Autodesk Inventor part; units mm, degrees
ref_plane "YZ Plane" through (0, 0, 0) normal (1, 0, 0) x (0, 1, 0)
ref_plane "XZ Plane" through (0, 0, 0) normal (0, 1, 0) x (-1, 0, 0)
ref_plane "XY Plane" through (0, 0, 0) normal (0, 0, 1) x (1, 0, 0)
sketch "Sketch1" plane through (0, 0, 0) normal (0, 0, 1) x (1, 0, 0)
  line L0 (-86, -45) -> (-46.4758, -45)
  arc A0 (-46.4758, -45) -> (-36.6914, -26.0526) centre (-46.4758, -33) ccw
  arc A1 (36.6914, -26.0526) -> (-36.6914, -26.0526) centre (0, 0) ccw
  arc A2 (36.6914, -26.0526) -> (46.4758, -45) centre (46.4758, -33) ccw
  line L1 (46.4758, -45) -> (86, -45)
  line L2 (0, -90.5431) -> (0, 67.5905) construction
  line L3 (-86, -61) -> (-46.4758, -61)
  arc A3 (-46.4758, -61) -> (-23.6456, -16.7895) centre (-46.4758, -33) ccw
  arc A4 (23.6456, -16.7895) -> (-23.6456, -16.7895) centre (0, 0) ccw
  arc A5 (23.6456, -16.7895) -> (46.4758, -61) centre (46.4758, -33) ccw
  line L4 (46.4758, -61) -> (86, -61)
  line L5 (-86, -45) -> (-86, -61)
  line L6 (86, -45) -> (86, -61)
  dimension "d0" = 90
  dimension "d1" = 12
  dimension "d2" = 45
  dimension "d3" = 172
  dimension "d4" = 16
extrude "Extrusion1" add sketch "Sketch1" along normal mid plane 70
sketch "Sketch2" plane through (0, 0, 0) normal (1, 0, 0) x (0, 1, 0)
  arc A0 (6.3443, 4) -> (6.3443, -4) centre (0, 0) ccw
  line L0 (6.3443, 4) -> (45, 4)
  line L1 (45, 4) -> (45, -4)
  line L2 (45, -4) -> (6.3443, -4)
  line L3 (45, -35) -> (45, 35)
  dimension "d7" = 15
  dimension "d8" = 8
extrude "Extrusion2" cut sketch "Sketch2" along normal through all both and the other way through all
sketch "Sketch3" plane through (0, 0, 0) normal (0, 0, 1) x (1, 0, 0)
  arc A0 (0, 73) -> (0, 17) centre (0, 45) ccw
  line L0 (-86, -61) -> (-46.4758, -61)
  line L1 (0, 73) -> (0, 17)
  arc A1 (44.5505, 6.3443) -> (-44.5505, 6.3443) centre (0, 0) ccw
  point P0 (-66.2379, -61)
  point P1 (0, 45)
  dimension "d11" = 28
  dimension "d12" = 106
revolve "Revolution1" cut sketch "Sketch3" angle 360 about axis through (0, 73, 0) along (0, -1, 0)
sketch "Sketch4" plane through (46.4758, -45, 35) normal (0, 1, 0) x (1, 0, 0)
  line L0 (18.5242, 19) -> (18.5242, 51) construction
  line L1 (12.5242, 19) -> (12.5242, 51)
  line L2 (24.5242, 51) -> (24.5242, 19)
  arc A0 (12.5242, 19) -> (24.5242, 19) centre (18.5242, 19) ccw
  arc A1 (24.5242, 51) -> (12.5242, 51) centre (18.5242, 51) ccw
  point P0 (-46.4758, 35)
  point P1 (18.5242, 35)
  dimension "d14" = 6
  dimension "d15" = 32
  dimension "d16" = 65
extrude "Extrusion3" cut sketch "Sketch4" against normal through all
mirror "Mirror1" about plane through (0, 0, 0) normal (1, 0, 0) of "Extrusion3"
fillet "Fillet1" radius 4 4 edges at (-86, -53, 35) (-86, -53, -35) (86, -53, 35) (86, -53, -35)
properties part number "Part013. Fulcrum" material "Steel, Carbon"
Geometry check sheet. Reference: the model listing, model coordinates, mm. A direction names the side the tool comes from. Give positions to 0.01 mm unless a question says otherwise; leave off trailing zeros. Loops run counter-clockwise (first coordinate to the right, second up) from the corner with the lowest first, then second, coordinate; pieces in that order, holes last. Notation, with made-up numbers: M -9,-33.5 L 32,-33.5 A6 ccw 32,-28.5 Z; hole C 53,-4 d6. An arc over 180 degrees is marked long. Write item = value, one per line.
(1) Material ranges on line 1 (X direction, y = -33, z = -12.5); line 2 (Z direction, x = -33, y = 0); line 3 (X direction, y = -54, z = -6), recorded low to high. Write a range as [from, to].
Answer below:
line_1 = [-34.48, -18.48], [18.48, 34.48]
line_2 = [-35, -7.5], [7.5, 35]
line_3 = [-86, -71], [-59, -27.96], [27.96, 59], [71, 86]
(2) Release check for a two-part mould opening along Z. For faces 1 (the face through (-58, -61, 0)), 2 (the face through (-31, 18, 4)), 3 (the face through (84.797, -53.112, -33.859)) record: released by +Z, released by -Z, zero draft, split by the parting line, or undercut.
Answer below:
face_1 = zero draft
face_2 = undercut
face_3 = released by -Z
(3) Sectioned sample at C-C, the plane z = 0. Record the cut outline in (x, y).
Answer below:
outline = M -86,-61 L -71,-61 L -71,-45 L -86,-45 Z; M -59,-61 L -46.48,-61 A28 ccw -23.65,-16.79 A29 cw -28.01,-7.5 L -44.37,-7.5 A45 ccw -36.69,-26.05 A12 cw -46.48,-45 L -59,-45 Z; M 23.65,-16.79 A28 ccw 46.48,-61 L 59,-61 L 59,-45 L 46.48,-45 A12 cw 36.69,-26.05 A45 ccw 44.37,-7.5 L 28.01,-7.5 A29 cw Z; M 71,-61 L 86,-61 L 86,-45 L 71,-45 Z
(4) Sectioned sample at A-A, the plane x = -65. Record the cut outline in (y, z).
Answer below:
outline = M -61,-35 L -45,-35 L -45,-22 L -61,-22 Z; M -61,22 L -45,22 L -45,35 L -61,35 Z
(5) Sectioned sample at B-B, the plane y = -51. Record the cut outline in (x, z).
Answer below:
outline = M -86,-31 A4 ccw -82,-35 L -25.03,-35 L -25.03,35 L -82,35 A4 ccw -86,31 Z; M 25.03,-35 L 82,-35 A4 ccw 86,-31 L 86,31 A4 ccw 82,35 L 25.03,35 Z; hole M -71,-16 A6 ccw -59,-16 L -59,16 A6 ccw -71,16 Z; hole M 59,-16 A6 ccw 71,-16 L 71,16 A6 ccw 59,16 Z
(6) Sectioned sample at D-D, the plane y = 0. Record the cut outline in (x, z).
Answer below:
outline = M -45,-35 L -29,-35 L -29,-7.5 L -45,-7.5 Z; M -45,7.5 L -29,7.5 L -29,35 L -45,35 Z; M 29,-35 L 45,-35 L 45,-7.5 L 29,-7.5 Z; M 29,7.5 L 45,7.5 L 45,35 L 29,35 Z
(7) Tool access check on faces 4 (the face through (-31, 18, -4)), 5 (the face through (-84.859, -53.112, -33.797)), 6 (the face through (-71, -53, 0)). Record the directions out of +Z, -Z, +X, -X, +Y, -Y that give a thin tool (end or side, any length) a straight path to the whole face; none if there is none.
Answer below:
face_4 = +X, -X, +Y
face_5 = -Z, -X, +Y, -Y
face_6 = +Y, -Y
(8) Gauge pin test, flat ends, axial feed: pin 1 Ø13.5 at (y, z) = (0, 0) entering from -X; pin 2 Ø4 at (y, z) = (-29, -11) entering from +X; pin 3 Ø8 at (y, z) = (-23, 27.5) entering from +X; pin 4 Ø6 at (x, z) = (6.5, -20) entering from -Y. Record the tip position at first contact, or that the pin passes through.
Answer below:
pin_1 = through
pin_2 = 36.08
pin_3 = 40.79
pin_4 = 27.4
